CAD build for the part. Positions are in the model's coordinates, mm. A direction names the side the tool comes from. Round coordinates to 2 decimals unless told otherwise and drop trailing zeros. Loops run counter-clockwise (first coordinate to the right, second up) from the corner with the lowest first, then second, coordinate; pieces in that order, holes last.
from build123d import *

# Parameters (mm, degrees)
BOX001027045148_W          = 4
BOX001027045148_H          = 3
BOX001027045148_DEPTH      = 20
BOX001027045148_ROLL_ANGLE = -29
BOX001027045147_W          = 4
BOX001027045147_H          = 3
BOX001027045147_DEPTH      = 20
BOX001027045147_ROLL_ANGLE = -29
CYLINDER203_R              = 1.7
CYLINDER203_DEPTH          = 30
CYLINDER203_PITCH_ANGLE    = 90
CYLINDER204_R              = 1.7
CYLINDER204_DEPTH          = 30
CYLINDER204_PITCH_ANGLE    = 90
CYLINDER202_R              = 1.7
CYLINDER202_DEPTH          = 30
CYLINDER202_PITCH_ANGLE    = 90
CYLINDER210_R              = 2
CYLINDER210_DEPTH          = 30
CYLINDER210_ROLL_ANGLE     = 13
CYLINDER209_R              = 2
CYLINDER209_DEPTH          = 30
CYLINDER209_ROLL_ANGLE     = -13
CYLINDER211_R              = 2
CYLINDER211_DEPTH          = 20
BOX001027045145_W          = 2.2
BOX001027045145_H          = 16
BOX001027045145_DEPTH      = 11
CHAMFER010_SIZE            = 7
CHAMFER011_SIZE            = 3
BOX001027045140_W          = 7
BOX001027045140_H          = 30
BOX001027045140_DEPTH      = 32
CHAMFER004_SIZE            = 4
CHAMFER012_SIZE            = 2


with BuildPart() as cube199:
    # Box001027045148 → Box001027045148 (new body)
    with BuildSketch(Plane.XY):
        with Locations((2, 1.5)):
            Rectangle(BOX001027045148_W, BOX001027045148_H)
    extrude(amount=BOX001027045148_DEPTH)


with BuildPart() as cube199_1:
    # Box001027045148 roll: moved
    add(cube199.part.rotate(Axis((0, 0, 0), (1, 0, 0)), BOX001027045148_ROLL_ANGLE))


with BuildPart() as cube199_2:
    # Box001027045148 placement: moved
    add(cube199_1.part.moved(Location((-2, 0, -2))))


with BuildPart() as part_mirroring002:
    # Part__Mirroring002: instance of Cube199
    add(cube199_2.part.mirror(Plane(origin=(0, 0, 0), x_dir=(1, 0, 0), z_dir=(0, 1, 0))))


with BuildPart() as split_holders001:
    # Box001027045147 → Box001027045147 (new body)
    with BuildSketch(Plane.XY):
        with Locations((2, 1.5)):
            Rectangle(BOX001027045147_W, BOX001027045147_H)
    extrude(amount=BOX001027045147_DEPTH)


with BuildPart() as split_holders001_1:
    # Box001027045147 roll: moved
    add(split_holders001.part.rotate(Axis((0, 0, 0), (1, 0, 0)), BOX001027045147_ROLL_ANGLE))


with BuildPart() as split_holders001_2:
    # Box001027045147 placement: moved
    add(split_holders001_1.part.moved(Location((-2, 0, -2))))

    # Fusion112099: union Part__Mirroring002
    add(part_mirroring002.part)


with BuildPart() as m3_clear_a:
    # Cylinder203 → Cylinder203 (new body)
    with BuildSketch(Plane.XY):
        Circle(CYLINDER203_R)
    extrude(amount=CYLINDER203_DEPTH)


with BuildPart() as m3_clear_a_1:
    # Cylinder203 pitch: moved
    add(m3_clear_a.part.rotate(Axis((0, 0, 0), (0, 1, 0)), CYLINDER203_PITCH_ANGLE))


with BuildPart() as m3_clear_a_2:
    # Cylinder203 placement: moved
    add(m3_clear_a_1.part.moved(Location((-15, 8, 0))))


with BuildPart() as m3_clear_b:
    # Cylinder204 → Cylinder204 (new body)
    with BuildSketch(Plane.XY):
        Circle(CYLINDER204_R)
    extrude(amount=CYLINDER204_DEPTH)


with BuildPart() as m3_clear_b_1:
    # Cylinder204 pitch: moved
    add(m3_clear_b.part.rotate(Axis((0, 0, 0), (0, 1, 0)), CYLINDER204_PITCH_ANGLE))


with BuildPart() as m3_clear_b_2:
    # Cylinder204 placement: moved
    add(m3_clear_b_1.part.moved(Location((-15, -8, 0))))


with BuildPart() as m3_clears:
    # Cylinder202 → Cylinder202 (new body)
    with BuildSketch(Plane.XY):
        Circle(CYLINDER202_R)
    extrude(amount=CYLINDER202_DEPTH)


with BuildPart() as m3_clears_1:
    # Cylinder202 pitch: moved
    add(m3_clears.part.rotate(Axis((0, 0, 0), (0, 1, 0)), CYLINDER202_PITCH_ANGLE))


with BuildPart() as m3_clears_2:
    # Cylinder202 placement: moved
    add(m3_clears_1.part.moved(Location((-15, 0, 24))))

    # Fusion112083: union M3-clear-a, M3-clear-b
    add(m3_clear_a_2.part)
    add(m3_clear_b_2.part)


with BuildPart() as cylinder210:
    # Cylinder210 → Cylinder210 (new body)
    with BuildSketch(Plane.XY):
        Circle(CYLINDER210_R)
    extrude(amount=CYLINDER210_DEPTH)


with BuildPart() as cylinder210_1:
    # Cylinder210 roll: moved
    add(cylinder210.part.rotate(Axis((0, 0, 0), (1, 0, 0)), CYLINDER210_ROLL_ANGLE))


with BuildPart() as cylinder210_2:
    # Cylinder210 placement: moved
    add(cylinder210_1.part.moved(Location((0, -2.249511, 9.743701))))


with BuildPart() as cylinder209:
    # Cylinder209 → Cylinder209 (new body)
    with BuildSketch(Plane.XY):
        Circle(CYLINDER209_R)
    extrude(amount=CYLINDER209_DEPTH)


with BuildPart() as cylinder209_1:
    # Cylinder209 roll: moved
    add(cylinder209.part.rotate(Axis((0, 0, 0), (1, 0, 0)), CYLINDER209_ROLL_ANGLE))


with BuildPart() as cylinder209_2:
    # Cylinder209 placement: moved
    add(cylinder209_1.part.moved(Location((0, 2.249511, 9.743701))))


with BuildPart() as cylinder243:
    # Cylinder211 → Cylinder211 (new body)
    with BuildSketch(Plane.XY.offset(-19)):
        Circle(CYLINDER211_R)
    extrude(amount=CYLINDER211_DEPTH)


with BuildPart() as y_top_m3:
    # Box001027045145 → Box001027045145 (new body)
    with BuildSketch(Plane(origin=(-1.1, -8, 0), x_dir=(1, 0, 0), z_dir=(0, 0, 1))):
        with Locations((1.1, 8)):
            Rectangle(BOX001027045145_W, BOX001027045145_H)
    extrude(amount=BOX001027045145_DEPTH)

    # Chamfer010
    chamfer010_edges = [y_top_m3.edges().sort_by_distance(p)[0] for p in [
        (0, -8, 0),
        (0, 8, 0),
    ]]
    chamfer(chamfer010_edges, length=CHAMFER010_SIZE)

    # Chamfer011
    chamfer011_edges = [y_top_m3.edges().sort_by_distance(p)[0] for p in [
        (0, -8, 7),
        (0, 8, 7),
    ]]
    chamfer(chamfer011_edges, length=CHAMFER011_SIZE)

    # Fusion112094: union Cylinder210, Cylinder209, Cylinder243
    add(cylinder210_2.part)
    add(cylinder209_2.part)
    add(cylinder243.part)

    # Fusion112100: union M3-clears
    add(m3_clears_2.part)


with BuildPart() as top:
    # Box001027045140 → Box001027045140 (new body)
    with BuildSketch(Plane(origin=(0, -15, -4), x_dir=(1, 0, 0), z_dir=(0, 0, 1))):
        with Locations((3.5, 15)):
            Rectangle(BOX001027045140_W, BOX001027045140_H)
    extrude(amount=BOX001027045140_DEPTH)

    # Chamfer004
    chamfer004_edges = [top.edges().sort_by_distance(p)[0] for p in [
        (3.5, -15, -4),
        (3.5, 15, -4),
    ]]
    chamfer(chamfer004_edges, length=CHAMFER004_SIZE)

    # Cut162: cut y-top-M3
    add(y_top_m3.part, mode=Mode.SUBTRACT)

    # Cut163: cut split-holders001
    add(split_holders001_2.part, mode=Mode.SUBTRACT)

    # Chamfer012
    chamfer012_edges = [top.edges().sort_by_distance(p)[0] for p in [
        (7, -8, 1.7),
        (7, 0, 25.7),
        (7, 8, 1.7),
    ]]
    chamfer(chamfer012_edges, length=CHAMFER012_SIZE)


with BuildPart() as top_1:
    # Chamfer012 placement: moved
    add(top.part.moved(Location((46, 0, 0))))


solid = top_1.part
Item 1: Cut at A-A (x = 50.5). List the corners of the cut face in (y, z), plus the area to 3 significant figures.
Verdict:
outline: (-15, 0) - (-11, -4) - (11, -4) - (15, 0) - (15, 28) - (-15, 28) - close; hole circle Ø3.4 at (-8, 0); hole circle Ø3.4 at (0, 24); hole circle Ø3.4 at (8, 0)
area: 917 mm2
Item 2: Cut at D-D (z = 4.5). List the corners of the cut face in (x, y).
Verdict:
outline: (46, -15) - (53, -15) - (53, 15) - (46, 15) - (46, 7.03) - (48, 7.03) - (48, 3.6) - (47.1, 3.6) - (47.1, -3.6) - (48, -3.6) - (48, -7.03) - (46, -7.03) - close
Item 3: Cut at B-B (x = 46.5). State how many separate pieces and enclosed holes the cut face has, plus the area to 3 significant figures.
Verdict:
separate pieces: 3
enclosed holes: 3
area: 562 mm2
Item 4: Flat gauge pin, fed straight in: P1, Ø2.5, axis at y = 8, z = 0, coming from the +X side. Where does the tip first touch, or does it go through?
Verdict:
P1: passes through
Item 5: Cut at C-C (z = 8). List the corners of the cut face in (x, y), plus the area to 3 significant figures.
Verdict:
outline: (46, -15) - (53, -15) - (53, 15) - (46, 15) - (46, 8.97) - (48, 8.97) - (48, 5.54) - (47.1, 5.54) - (47.1, -5.54) - (48, -5.54) - (48, -8.97) - (46, -8.97) - close
area: 184 mm2
Item 6: Mould opens along Y. For faces 4 (the flat face through (49, -13, -2)), 5 (the flat face through (47.1, 0, 7)), 6 (the flat face through (46, 0, 21)) say: released by +Y, released by -Y, zero draft, split by the parting line, or undercut.
Verdict:
face 4: released by -Y
face 5: undercut
face 6: zero draft
Item 7: 3-axis set-ups, long thin cutter, end or side, ignore diameter. For faces 1 (the flat face through (46.5, 0, 11)), 2 (the flat face through (49, 13, -2)), 3 (the flat face through (47.21, -1.91, -3.06)): which of +Z, -Z, +X, -X, +Y, -Y reach the whole face in a straight line?
Verdict:
face 1: -Z, -X
face 2: -Z, +X, -X, +Y
face 3: -X
Item 8: Wall check: L1, parallel to Y at x = 46.5, z = 24; L2, parallel to Z at x = 49.05, y = -8; L3, parallel to Z at x = 47.5, y = 8. Give the ranges that are in metal, low to high.
Verdict:
L1: y = -15 to -7.53, -3.55 to -1.7, 1.7 to 3.55, 7.53 to 15
L2: z = -4 to -1.7, 1.7 to 28
L3: z = -4 to -1.7, 1.7 to 6.24, 12.43 to 28
